Build history of the part. All positions in model axes, mm. Face numbers are marked on the shaded views. A direction names the side the tool comes from. Give positions to 0.01 mm unless a question says otherwise; leave off trailing zeros. Order: outer loops, then holes, each group sorted by start corner. A loop starts at its lowest first (then second) coordinate and runs counter-clockwise, first axis right, second up. Notation, with made-up numbers: (9, 26) - (19, 26) arc R10 cw to (19, 30) - close; hole circle Ø9 at (41, 10). An arc over 180 degrees is marked (long way). Write each question's results on one line, items separated by ' | '. Start each with the question number.
1) Cut at A-A on x = 30. List the corners of the cut face in (y, z), plus the area to 3 significant figures.
2) Tool access for the marked faces 1, 2, 3 and 4: list every direction of +Z, -Z, +X, -X, +Y, -Y with a clear straight run to the whole face (end or side of a thin tool).
3) Drill centre lines: line 1 along Z through (x, y) = (31, 13); line 2 along Z through (x, y) = (30, 4); line 3 along X through (y, z) = (4.75, 140). Where is each one in solid material? Low to high. Write a range as from..to.
4) Drop flat-ended pins along their axis: pin 1 Ø4 at (x, z) = (42.9, 152.9) entering from +Y; pin 2 Ø5 at (y, z) = (23.5, 92.5) entering from +X; pin 3 Ø12 at (y, z) = (23.5, 30.5) entering from +X. Give the stop position or say it passes through.
5) Cut at B-B on z = 45. List the corners of the cut face in (x, y), plus the area to 3 significant figures.
6) Two-plate mould, pull along X, no slides. Class the marked faces 5, 6 and 7: +X half, -X half, draft (parallel to the pull), parting line (faces both ways), or undercut.
7) Cut at C-C on y = 14. State how many separate pieces and enclosed holes the cut face has, plus the area to 3 significant figures.
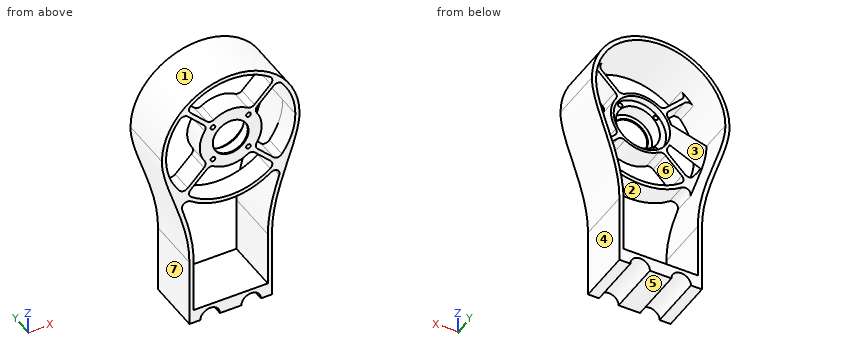
from build123d import *

# Parameters (mm, degrees)
EXTRUDE_1_DEPTH            = 40
CUT_EXTRUDE_1_DEPTH        = 41.0000001
SKETCH_3_R                 = 22.5
SKETCH_3_R_2               = 13
EXTRUDE_2_DEPTH            = 16
SKETCH_4_R                 = 20.5
CUT_EXTRUDE_2_DEPTH        = 5
SKETCH_5_R                 = 16
CUT_EXTRUDE_3_DEPTH        = 10
SKETCH_7_W                 = 1.7
SKETCH_7_H                 = 11
HOLE_WIZARD_M31_AT_2_COUNT = 2
HOLE_WIZARD_M31_AT_2_PITCH = 25.809397513
HOLE_WIZARD_M31_AT_3_COUNT = 2
HOLE_WIZARD_M31_AT_3_PITCH = 36.5
HOLE_WIZARD_M31_AT_4_COUNT = 2
HOLE_WIZARD_M31_AT_4_PITCH = 25.809397513
EXTRUDE_3_DEPTH            = 16
EXTRUDE_4_DEPTH            = 16
FILLET_1_R                 = 4
FILLET_2_R                 = 4
EXTRUDE_5_DEPTH            = 40


with BuildPart() as part:
    # Sketch 1 → Extrude 1 (new body)
    with BuildSketch(Plane(origin=(0, 0, 0), x_dir=(1, 0, 0), z_dir=(0, 1, 0))):
        with BuildLine():
            Line((0, 0), (8, 0))
            ThreePointArc((8, 0), (15.1, -7.1), (22.2, 0))
            Line((22.2, 0), (37.8, 0))
            ThreePointArc((37.8, 0), (44.9, -7.1), (52, 0))
            Line((52, 0), (60, 0))
            Line((60, 0), (60, -50))
            add(Edge.make_bspline(
                [(60, -50), (60, -86.116353651), (80.160728995, -116.642608399), (80, -140)],
                knots=[0, 0, 0, 0, 1, 1, 1, 1], degree=3))
            ThreePointArc((80, -140), (30, -190), (-20, -140))
            add(Edge.make_bspline(
                [(0, -50), (0, -86.116353651), (-20.160728995, -116.642608399), (-20, -140)],
                knots=[0, 0, 0, 0, 1, 1, 1, 1], degree=3))
            Line((0, -50), (0, 0))
        make_face()
    extrude(amount=EXTRUDE_1_DEPTH)

    # Sketch 2 → Cut-Extrude 1 (cut, through all)
    with BuildSketch(Plane.XZ):
        with BuildLine():
            Line((3, 50), (3, 3))
            Line((3, 3), (5.455830777, 3))
            ThreePointArc((5.455830777, 3), (15.1, 10.1), (24.744169223, 3))
            Line((24.744169223, 3), (35.255830777, 3))
            ThreePointArc((35.255830777, 3), (44.9, 10.1), (54.544169223, 3))
            Line((54.544169223, 3), (57, 3))
            Line((57, 3), (57, 50))
            add(Edge.make_bspline(
                [(57, 50), (57, 51.157609129), (57.040606582, 53.481410198), (57.273704219, 58.056259254), (57.830047707, 63.685631551), (58.858223783, 70.278683586), (60.625819875, 78.854483127), (63.422404864, 89.162496802), (67.223313935, 100.856350391), (70.98262402, 111.850711206), (73.680271867, 120.398992166), (75.344252207, 126.83842419), (76.290135947, 131.459638595), (76.783312256, 135.122784785), (76.977813987, 137.947550146), (77.004716082, 139.304329707), (76.999998901, 139.989837839)],
                knots=[0, 0, 0, 0, 0.031254674, 0.062509349, 0.125018697, 0.187528046, 0.250037394, 0.375056092, 0.500074789, 0.625093486, 0.750112183, 0.812621532, 0.87513088, 0.937640229, 0.968894903, 1.000149578, 1.000149578, 1.000149578, 1.000149578], degree=3))
            ThreePointArc((76.999998901, 139.989837839), (30, 187), (-16.999998901, 139.989837839))
            add(Edge.make_bspline(
                [(-16.999998901, 139.989837839), (-17.004716082, 139.304329707), (-16.977813987, 137.947550146), (-16.783312256, 135.122784785), (-16.290135947, 131.459638595), (-15.344252207, 126.83842419), (-13.680271867, 120.398992166), (-10.98262402, 111.850711206), (-7.223313935, 100.856350391), (-3.422404864, 89.162496802), (-0.625819875, 78.854483127), (1.141776217, 70.278683586), (2.169952293, 63.685631551), (2.726295781, 58.056259254), (2.959393418, 53.481410198), (3, 51.157609129), (3, 50)],
                knots=[-0.000149578, -0.000149578, -0.000149578, -0.000149578, 0.031105097, 0.062359771, 0.12486912, 0.187378468, 0.249887817, 0.374906514, 0.499925211, 0.624943908, 0.749962606, 0.812471954, 0.874981303, 0.937490651, 0.968745326, 1, 1, 1, 1], degree=3))
        make_face()
    extrude(amount=-CUT_EXTRUDE_1_DEPTH, mode=Mode.SUBTRACT)

    # Sketch 9 → Extrude 3 (add)
    with BuildSketch(Plane.XZ):
        with BuildLine():
            ThreePointArc((-10.590299222, 110.803637057), (30, 90), (70.590299222, 110.803637057))
            add(Edge.make_bspline(
                [(70.590299222, 110.803637057), (70.692686494, 111.112669843), (71.968099867, 114.973477738), (73.680271867, 120.398992166), (75.344252207, 126.83842419), (76.290135947, 131.459638595), (76.783312256, 135.122784785), (76.977813987, 137.947550146), (77.004716082, 139.304329707), (76.999998901, 139.989837839)],
                knots=[0.614251021, 0.614251021, 0.614251021, 0.614251021, 0.625093486, 0.750112183, 0.812621532, 0.87513088, 0.937640229, 0.968894903, 1.000149578, 1.000149578, 1.000149578, 1.000149578], degree=3))
            ThreePointArc((76.999998901, 139.989837839), (30, 93), (-16.999998901, 139.989837839))
            add(Edge.make_bspline(
                [(-16.999998901, 139.989837839), (-17.004716082, 139.304329707), (-16.977813987, 137.947550146), (-16.783312256, 135.122784785), (-16.290135947, 131.459638595), (-15.344252207, 126.83842419), (-13.680271867, 120.398992166), (-11.968099867, 114.973477738), (-10.692686494, 111.112669843), (-10.590299222, 110.803637057)],
                knots=[-0.000149578, -0.000149578, -0.000149578, -0.000149578, 0.031105097, 0.062359771, 0.12486912, 0.187378468, 0.249887817, 0.374906514, 0.385748979, 0.385748979, 0.385748979, 0.385748979], degree=3))
        make_face()
    extrude(amount=-EXTRUDE_3_DEPTH)



with BuildPart() as body_2:
    # Sketch 3 → Extrude 2 (new body)
    with BuildSketch(Plane.XZ):
        with Locations((30, 140)):
            Circle(SKETCH_3_R)
        with Locations((30, 140)):
            Circle(SKETCH_3_R_2, mode=Mode.SUBTRACT)
    extrude(amount=-EXTRUDE_2_DEPTH)

    # Sketch 4 → Cut-Extrude 2 (cut)
    with BuildSketch(Plane(origin=(0, 16, 0), x_dir=(1, 0, 0), z_dir=(0, 1, 0))):
        with Locations((30, -140)):
            Circle(SKETCH_4_R)
    extrude(amount=-CUT_EXTRUDE_2_DEPTH, mode=Mode.SUBTRACT)

    # Sketch 5 → Cut-Extrude 3 (cut)
    with BuildSketch(Plane(origin=(0, 11, 0), x_dir=(1, 0, 0), z_dir=(0, 1, 0))):
        with Locations((30, -140)):
            Circle(SKETCH_5_R)
    extrude(amount=-CUT_EXTRUDE_3_DEPTH, mode=Mode.SUBTRACT)

    # Sketch 7 → Hole Wizard M31 (revolve, cut)
    with BuildSketch(Plane(origin=(17.095301243, 11, 127.095301243), x_dir=(0, 0, 1), z_dir=(1, 0, 0))):
        with Locations((0.85, 5.5)):
            Rectangle(SKETCH_7_W, SKETCH_7_H)
    hole_wizard_m31 = revolve(axis=Axis((17.095301243, 17.35, 127.095301243), (0, -1, 0)), mode=Mode.SUBTRACT)

    # Hole Wizard M31 at 2: Hole Wizard M31 ×2
    with Locations(*[(i * HOLE_WIZARD_M31_AT_2_PITCH, 0, 0) for i in range(1, HOLE_WIZARD_M31_AT_2_COUNT)]):
        add(hole_wizard_m31, mode=Mode.SUBTRACT)

    # Hole Wizard M31 at 3: Hole Wizard M31 ×2
    with Locations(*[Vector(0.707106781, 0, 0.707106781) * (i * HOLE_WIZARD_M31_AT_3_PITCH) for i in range(1, HOLE_WIZARD_M31_AT_3_COUNT)]):
        add(hole_wizard_m31, mode=Mode.SUBTRACT)

    # Hole Wizard M31 at 4: Hole Wizard M31 ×2
    with Locations(*[(0, 0, i * HOLE_WIZARD_M31_AT_4_PITCH) for i in range(1, HOLE_WIZARD_M31_AT_4_COUNT)]):
        add(hole_wizard_m31, mode=Mode.SUBTRACT)


with BuildPart() as part_1:
    add(part.part)

    add(body_2.part)  # Extrude 4 merges body 2
    # Sketch 10 → Extrude 4 (add)
    with BuildSketch(Plane.XZ):
        with BuildLine():
            Line((13.061629364, 154.810185691), (-4.284701087, 172.149016647))
            ThreePointArc((-4.284701087, 172.149016647), (-3.241203672, 173.226832206), (-2.163839457, 174.270795605))
            Line((-2.163839457, 174.270795605), (15.182490994, 156.931964648))
            ThreePointArc((15.182490994, 156.931964648), (14.086657817, 155.906462226), (13.061629364, 154.810185691))
        make_face()
        with BuildLine():
            Line((15.189814309, 123.061629364), (-2.149016647, 105.715298913))
            ThreePointArc((-2.149016647, 105.715298913), (-3.226832206, 106.758796328), (-4.270795605, 107.836160543))
            Line((-4.270795605, 107.836160543), (13.068035352, 125.182490994))
            ThreePointArc((13.068035352, 125.182490994), (14.093537774, 124.086657817), (15.189814309, 123.061629364))
        make_face()
        with BuildLine():
            Line((44.810185691, 156.938370636), (62.149016647, 174.284701087))
            ThreePointArc((62.149016647, 174.284701087), (63.226832206, 173.241203672), (64.270795605, 172.163839457))
            Line((64.270795605, 172.163839457), (46.931964648, 154.817509006))
            ThreePointArc((46.931964648, 154.817509006), (45.906462226, 155.913342183), (44.810185691, 156.938370636))
        make_face()
        with BuildLine():
            Line((46.938370636, 125.189814309), (64.284701087, 107.850983353))
            ThreePointArc((64.284701087, 107.850983353), (63.241203672, 106.773167794), (62.163839457, 105.729204395))
            Line((62.163839457, 105.729204395), (44.817509006, 123.068035352))
            ThreePointArc((44.817509006, 123.068035352), (45.913342183, 124.093537774), (46.938370636, 125.189814309))
        make_face()
    extrude(amount=-EXTRUDE_4_DEPTH)

    # Fillet 1
    fillet_1_edges = [part_1.edges().sort_by_distance(p)[0] for p in [
        (70.590299222, 8, 110.803637057),
        (-10.590299222, 8, 110.803637057),
    ]]
    fillet(fillet_1_edges, radius=FILLET_1_R)

    # Fillet 2
    fillet_2_edges = [part_1.edges().sort_by_distance(p)[0] for p in [
        (-4.284701087, 8, 172.149016647),
        (-2.163839457, 8, 174.270795605),
        (15.182490994, 8, 156.931964648),
        (13.061629364, 8, 154.810185691),
        (62.149016647, 8, 174.284701087),
        (64.270795605, 8, 172.163839457),
        (46.931964648, 8, 154.817509006),
        (44.810185691, 8, 156.938370636),
        (64.284701087, 8, 107.850983353),
        (62.163839457, 8, 105.729204395),
        (44.817509006, 8, 123.068035352),
        (46.938370636, 8, 125.189814309),
        (-2.149016647, 8, 105.715298913),
        (-4.270795605, 8, 107.836160543),
        (13.068035352, 8, 125.182490994),
        (15.189814309, 8, 123.061629364),
    ]]
    fillet(fillet_2_edges, radius=FILLET_2_R)

    # Sketch 11 → Extrude 5 (add, through all)
    with BuildSketch(Plane(origin=(0, 40, 0), x_dir=(1, 0, 0), z_dir=(0, 1, 0))):
        with BuildLine():
            ThreePointArc((24.744169223, -3), (21.087904475, -8.133572401), (15.1, -10.1))
            Line((15.1, -10.1), (44.9, -10.1))
            ThreePointArc((44.9, -10.1), (38.912095525, -8.133572401), (35.255830777, -3))
            Line((35.255830777, -3), (24.744169223, -3))
        make_face()
        with BuildLine():
            ThreePointArc((54.544169223, -3), (50.887904475, -8.133572401), (44.9, -10.1))
            Line((44.9, -10.1), (57, -10.1))
            Line((57, -10.1), (57, -3))
            Line((57, -3), (54.544169223, -3))
        make_face()
        with BuildLine():
            Line((3, -3), (3, -10.1))
            Line((3, -10.1), (15.1, -10.1))
            ThreePointArc((15.1, -10.1), (9.112095525, -8.133572401), (5.455830777, -3))
            Line((5.455830777, -3), (3, -3))
        make_face()
    extrude(amount=-EXTRUDE_5_DEPTH)


solid = part_1.part
Results:
1) outline: (0, 0) - (40, 0) - (40, 10.1) - (0, 10.1) - close; (0, 90) - (16, 90) - (16, 93) - (0, 93) - close; (0, 117.5) - (16, 117.5) - (16, 119.5) - (11, 119.5) - (11, 124) - (1, 124) - (1, 127) - (0, 127) - close; (0, 153) - (1, 153) - (1, 156) - (11, 156) - (11, 160.5) - (16, 160.5) - (16, 162.5) - (0, 162.5) - close; (0, 187) - (40, 187) - (40, 190) - (0, 190) - close | area: 741 mm^2
2) face 1: +Z, +Y, -Y | face 2: +Y, -Y | face 3: +Y | face 4: -Z, +X, +Y, -Y
3) line 1: 0..10.1, 90.01..93.01, 117.52..119.52, 160.48..162.48, 186.99..189.99 | line 2: 0..10.1, 90..93, 117.5..124, 156..162.5, 187..190 | line 3: -20..-17, 7.5..14, 46..52.5, 77..80
4) pin 1: y = 11 | pin 2: x = 68.49 | pin 3: x = 60
5) outline: (0, 0) - (3, 0) - (3, 40) - (0, 40) - close; (57, 0) - (60, 0) - (60, 40) - (57, 40) - close | area: 240 mm^2
6) face 5: draft | face 6: undercut | face 7: -X half
7) separate pieces: 1 | enclosed holes: 6 | area: 2,710 mm^2
